```python
from build123d import *

# Parameters (mm, degrees)
SKETCH1_R           = 8.5
BOSS_EXTRUDE1_DEPTH = 20


with BuildPart() as part:
    # Sketch1 → Boss-Extrude1 (new body)
    with BuildSketch(Plane.XY):
        Circle(SKETCH1_R)
        with BuildLine():
            Line((-1.463336561, 6.256639256), (-0.593931236, 4.646135995))
            ThreePointArc((-0.593931236, 4.646135995), (-0.474689485, 4.525877032), (-0.309320024, 4.489356426))
            ThreePointArc((-0.309320024, 4.489356426), (0, 4.5), (0.309320024, 4.489356426))
            ThreePointArc((0.309320024, 4.489356426), (0.474689485, 4.525877032), (0.593931236, 4.646135995))
            Line((0.593931236, 4.646135995), (1.463336561, 6.256639256))
            ThreePointArc((1.463336561, 6.256639256), (1.510970427, 6.300627973), (1.575572767, 6.30615338))
            ThreePointArc((1.575572767, 6.30615338), (1.682323793, 6.278517871), (1.788590648, 6.249075411))
            ThreePointArc((1.788590648, 6.249075411), (1.841775212, 6.211989098), (1.861032992, 6.150076818))
            Line((1.861032992, 6.150076818), (1.808708459, 4.320637419))
            ThreePointArc((1.808708459, 4.320637419), (1.851845362, 4.156869226), (1.976799214, 4.042556724))
            ThreePointArc((1.976799214, 4.042556724), (2.25, 3.897114317), (2.512557212, 3.7332367))
            ThreePointArc((2.512557212, 3.7332367), (2.674031669, 3.682179741), (2.837427536, 3.726706183))
            Line((2.837427536, 3.726706183), (4.395606264, 4.686740257))
            ThreePointArc((4.395606264, 4.686740257), (4.458852761, 4.70101867), (4.517562732, 4.673502644))
            ThreePointArc((4.517562732, 4.673502644), (4.596194078, 4.596194078), (4.673502644, 4.517562732))
            ThreePointArc((4.673502644, 4.517562732), (4.70101867, 4.458852761), (4.686740257, 4.395606264))
            Line((4.686740257, 4.395606264), (3.726706183, 2.837427536))
            ThreePointArc((3.726706183, 2.837427536), (3.682179741, 2.674031669), (3.7332367, 2.512557212))
            ThreePointArc((3.7332367, 2.512557212), (3.897114317, 2.25), (4.042556724, 1.976799214))
            ThreePointArc((4.042556724, 1.976799214), (4.156869226, 1.851845362), (4.320637419, 1.808708459))
            Line((4.320637419, 1.808708459), (6.150076818, 1.861032992))
            ThreePointArc((6.150076818, 1.861032992), (6.211989098, 1.841775212), (6.249075411, 1.788590648))
            ThreePointArc((6.249075411, 1.788590648), (6.278517871, 1.682323793), (6.30615338, 1.575572767))
            ThreePointArc((6.30615338, 1.575572767), (6.300627973, 1.510970427), (6.256639256, 1.463336561))
            Line((6.256639256, 1.463336561), (4.646135995, 0.593931236))
            ThreePointArc((4.646135995, 0.593931236), (4.525877032, 0.474689485), (4.489356426, 0.309320024))
            ThreePointArc((4.489356426, 0.309320024), (4.5, 0), (4.489356426, -0.309320024))
            ThreePointArc((4.489356426, -0.309320024), (4.525877032, -0.474689485), (4.646135995, -0.593931236))
            Line((4.646135995, -0.593931236), (6.256639256, -1.463336561))
            ThreePointArc((6.256639256, -1.463336561), (6.300627973, -1.510970427), (6.30615338, -1.575572767))
            ThreePointArc((6.30615338, -1.575572767), (6.278517871, -1.682323793), (6.249075411, -1.788590648))
            ThreePointArc((6.249075411, -1.788590648), (6.211989098, -1.841775212), (6.150076818, -1.861032992))
            Line((6.150076818, -1.861032992), (4.320637419, -1.808708459))
            ThreePointArc((4.320637419, -1.808708459), (4.156869226, -1.851845362), (4.042556724, -1.976799214))
            ThreePointArc((4.042556724, -1.976799214), (3.897114317, -2.25), (3.7332367, -2.512557212))
            ThreePointArc((3.7332367, -2.512557212), (3.682179741, -2.674031669), (3.726706183, -2.837427536))
            Line((3.726706183, -2.837427536), (4.686740257, -4.395606264))
            ThreePointArc((4.686740257, -4.395606264), (4.70101867, -4.458852761), (4.673502644, -4.517562732))
            ThreePointArc((4.673502644, -4.517562732), (4.596194078, -4.596194078), (4.517562732, -4.673502644))
            ThreePointArc((4.517562732, -4.673502644), (4.458852761, -4.70101867), (4.395606264, -4.686740257))
            Line((4.395606264, -4.686740257), (2.837427536, -3.726706183))
            ThreePointArc((2.837427536, -3.726706183), (2.674031669, -3.682179741), (2.512557212, -3.7332367))
            ThreePointArc((2.512557212, -3.7332367), (2.25, -3.897114317), (1.976799214, -4.042556724))
            ThreePointArc((1.976799214, -4.042556724), (1.851845362, -4.156869226), (1.808708459, -4.320637419))
            Line((1.808708459, -4.320637419), (1.861032992, -6.150076818))
            ThreePointArc((1.861032992, -6.150076818), (1.841775212, -6.211989098), (1.788590648, -6.249075411))
            ThreePointArc((1.788590648, -6.249075411), (1.682323793, -6.278517871), (1.575572767, -6.30615338))
            ThreePointArc((1.575572767, -6.30615338), (1.510970427, -6.300627973), (1.463336561, -6.256639256))
            Line((1.463336561, -6.256639256), (0.593931236, -4.646135995))
            ThreePointArc((0.593931236, -4.646135995), (0.474689485, -4.525877032), (0.309320024, -4.489356426))
            ThreePointArc((0.309320024, -4.489356426), (0, -4.5), (-0.309320024, -4.489356426))
            ThreePointArc((-0.309320024, -4.489356426), (-0.474689485, -4.525877032), (-0.593931236, -4.646135995))
            Line((-0.593931236, -4.646135995), (-1.463336561, -6.256639256))
            ThreePointArc((-1.463336561, -6.256639256), (-1.510970427, -6.300627973), (-1.575572767, -6.30615338))
            ThreePointArc((-1.575572767, -6.30615338), (-1.682323793, -6.278517871), (-1.788590648, -6.249075411))
            ThreePointArc((-1.788590648, -6.249075411), (-1.841775212, -6.211989098), (-1.861032992, -6.150076818))
            Line((-1.861032992, -6.150076818), (-1.808708459, -4.320637419))
            ThreePointArc((-1.808708459, -4.320637419), (-1.851845362, -4.156869226), (-1.976799214, -4.042556724))
            ThreePointArc((-1.976799214, -4.042556724), (-2.25, -3.897114317), (-2.512557212, -3.7332367))
            ThreePointArc((-2.512557212, -3.7332367), (-2.674031669, -3.682179741), (-2.837427536, -3.726706183))
            Line((-2.837427536, -3.726706183), (-4.395606264, -4.686740257))
            ThreePointArc((-4.395606264, -4.686740257), (-4.458852761, -4.70101867), (-4.517562732, -4.673502644))
            ThreePointArc((-4.517562732, -4.673502644), (-4.596194078, -4.596194078), (-4.673502644, -4.517562732))
            ThreePointArc((-4.673502644, -4.517562732), (-4.70101867, -4.458852761), (-4.686740257, -4.395606264))
            Line((-4.686740257, -4.395606264), (-3.726706183, -2.837427536))
            ThreePointArc((-3.726706183, -2.837427536), (-3.682179741, -2.674031669), (-3.7332367, -2.512557212))
            ThreePointArc((-3.7332367, -2.512557212), (-3.897114317, -2.25), (-4.042556724, -1.976799214))
            ThreePointArc((-4.042556724, -1.976799214), (-4.156869226, -1.851845362), (-4.320637419, -1.808708459))
            Line((-4.320637419, -1.808708459), (-6.150076818, -1.861032992))
            ThreePointArc((-6.150076818, -1.861032992), (-6.211989098, -1.841775212), (-6.249075411, -1.788590648))
            ThreePointArc((-6.249075411, -1.788590648), (-6.278517871, -1.682323793), (-6.30615338, -1.575572767))
            ThreePointArc((-6.30615338, -1.575572767), (-6.300627973, -1.510970427), (-6.256639256, -1.463336561))
            Line((-6.256639256, -1.463336561), (-4.646135995, -0.593931236))
            ThreePointArc((-4.646135995, -0.593931236), (-4.525877032, -0.474689485), (-4.489356426, -0.309320024))
            ThreePointArc((-4.489356426, -0.309320024), (-4.5, 0), (-4.489356426, 0.309320024))
            ThreePointArc((-4.489356426, 0.309320024), (-4.525877032, 0.474689485), (-4.646135995, 0.593931236))
            Line((-4.646135995, 0.593931236), (-6.256639256, 1.463336561))
            ThreePointArc((-6.256639256, 1.463336561), (-6.300627973, 1.510970427), (-6.30615338, 1.575572767))
            ThreePointArc((-6.30615338, 1.575572767), (-6.278517871, 1.682323793), (-6.249075411, 1.788590648))
            ThreePointArc((-6.249075411, 1.788590648), (-6.211989098, 1.841775212), (-6.150076818, 1.861032992))
            Line((-6.150076818, 1.861032992), (-4.320637419, 1.808708459))
            ThreePointArc((-4.320637419, 1.808708459), (-4.156869226, 1.851845362), (-4.042556724, 1.976799214))
            ThreePointArc((-4.042556724, 1.976799214), (-3.897114317, 2.25), (-3.7332367, 2.512557212))
            ThreePointArc((-3.7332367, 2.512557212), (-3.682179741, 2.674031669), (-3.726706183, 2.837427536))
            Line((-3.726706183, 2.837427536), (-4.686740257, 4.395606264))
            ThreePointArc((-4.686740257, 4.395606264), (-4.70101867, 4.458852761), (-4.673502644, 4.517562732))
            ThreePointArc((-4.673502644, 4.517562732), (-4.596194078, 4.596194078), (-4.517562732, 4.673502644))
            ThreePointArc((-4.517562732, 4.673502644), (-4.458852761, 4.70101867), (-4.395606264, 4.686740257))
            Line((-4.395606264, 4.686740257), (-2.837427536, 3.726706183))
            ThreePointArc((-2.837427536, 3.726706183), (-2.674031669, 3.682179741), (-2.512557212, 3.7332367))
            ThreePointArc((-2.512557212, 3.7332367), (-2.25, 3.897114317), (-1.976799214, 4.042556724))
            ThreePointArc((-1.976799214, 4.042556724), (-1.851845362, 4.156869226), (-1.808708459, 4.320637419))
            Line((-1.808708459, 4.320637419), (-1.861032992, 6.150076818))
            ThreePointArc((-1.861032992, 6.150076818), (-1.841775212, 6.211989098), (-1.788590648, 6.249075411))
            ThreePointArc((-1.788590648, 6.249075411), (-1.682323793, 6.278517871), (-1.575572767, 6.30615338))
            ThreePointArc((-1.575572767, 6.30615338), (-1.510970427, 6.300627973), (-1.463336561, 6.256639256))
        make_face(mode=Mode.SUBTRACT)
    extrude(amount=BOSS_EXTRUDE1_DEPTH)


solid = part.part
```
Geometry: final body of the model. Coordinates: model frame, mm. Round coordinates to 2 decimals unless told otherwise and drop trailing zeros. Write each loop counter-clockwise with the first axis right and the second up, starting at its lowest first coordinate (ties: lowest second). Pieces come first, ordered by that corner, then holes. Notation, with made-up numbers: M 49,64 L 103,64 A24 cw 103,86 Z; hole C 42,34.25 d4. An arc over 180 degrees is marked long. Answer in a Markdown table with one row per item. Add a question column.
(1) Draft query along X for faces 1 (the face through (3.627, -4.213, 9.86)), 2 (the face through (0, -6, 0)). Return one class per face: pulls with the +X half, pulls with the -X half, needs draft (parallel to the pull), parting line crosses it, or undercut.
(2) Cut plane C-C, the plane y = -5. Return the cut outline in (x, z).
(3) Cut plane D-D, the plane y = 7.25. Return the cut outline in (x, z).
(4) Ray query, L1, parallel to Y at x = 3.75, z = 10.5; L2, parallel to Y at x = -5.25, z = 16.5; L3, parallel to Y at x = 6, z = 8.75. Return the intervals inside material, ascending.
(5) Contact query for flat-ended pins moving along their axis: pin 1 (1 mm diameter, centred on y = -5, z = 9.5, fed in from -X); pin 2 (4 mm diameter, centred on x = -4, z = 11.5, fed in from -Y); pin 3 (1 mm diameter, centred on x = -6, z = 11, fed in from -Y). Output: stop coordinate, or through.
(6) Cut plane A-A, the plane x = 0. Return the cut outline in (y, z).
Established:
| question | item | result |
|---|---|---|
| 1 | face 1 | undercut |
| 1 | face 2 | needs draft |
| 2 | outline | M -6.87,0 L -1.83,0 L -1.83,20 L -6.87,20 Z; M -0.78,0 L 0.78,0 L 0.78,20 L -0.78,20 Z; M 1.83,0 L 6.87,0 L 6.87,20 L 1.83,20 Z |
| 3 | outline | M -4.44,0 L 4.44,0 L 4.44,20 L -4.44,20 Z |
| 4 | L1 | -7.63 to -4.29, -2.88 to -2.49, 2.49 to 2.88, 4.29 to 7.63 |
| 4 | L2 | -6.68 to -1.84, -0.92 to 0.92, 1.84 to 6.68 |
| 4 | L3 | -6.02 to -1.86, -1.32 to 1.32, 1.86 to 6.02 |
| 5 | pin 1 | x = -7.21 |
| 5 | pin 2 | y = -8.26 |
| 5 | pin 3 | y = -6.48 |
| 6 | outline | M -8.5,0 L -4.5,0 L -4.5,20 L -8.5,20 Z; M 4.5,0 L 8.5,0 L 8.5,20 L 4.5,20 Z |
